Can you work these out from the model? Positions are in its coordinate system, mm. Give positions to 0.01 mm unless a question says otherwise; leave off trailing zeros. Write each loop counter-clockwise with the first axis right and the second up, starting at its lowest first coordinate (ties: lowest second). Pieces come first, ordered by that corner, then holes. Notation, with made-up numbers: (45.5, -4.75) -> (69.5, -4.75) arc R24 cw to (69.5, 31.25) -> close; hole circle Ø3 at (11.5, 38). An arc over 180 degrees is marked (long way). One line per item, written item: value.
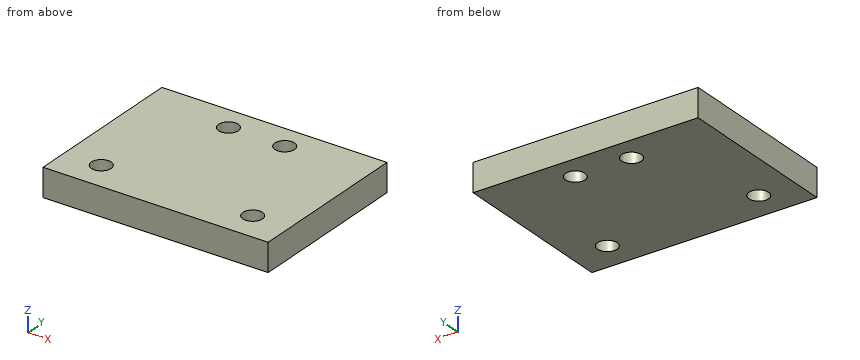
from build123d import *

# Parameters (mm, degrees)
SKETCH1_W           = 40
SKETCH1_H           = 30
SKETCH1_R           = 1.75
BOSS_EXTRUDE1_DEPTH = 5


with BuildPart() as part:
    # Sketch1 → Boss-Extrude1 (new body)
    with BuildSketch(Plane.XY):
        with Locations((20, 15)):
            Rectangle(SKETCH1_W, SKETCH1_H)
        with Locations((15, 25.5)):
            Circle(SKETCH1_R, mode=Mode.SUBTRACT)
        with Locations(Location((25, 25.5, 0), (0, 0, 180))):
            Circle(SKETCH1_R, mode=Mode.SUBTRACT)
        with Locations((6.55, 5.4)):
            Circle(SKETCH1_R, mode=Mode.SUBTRACT)
        with Locations(Location((33.45, 5.4, 0), (0, 0, 180))):
            Circle(SKETCH1_R, mode=Mode.SUBTRACT)
    extrude(amount=-BOSS_EXTRUDE1_DEPTH)


solid = part.part
1) If we section it at B-B (x = 33.45): Write out the boundary of the cut face in (y, z).
Answer list:
outline: (0, -5) -> (3.65, -5) -> (3.65, 0) -> (0, 0) -> close; (7.15, -5) -> (30, -5) -> (30, 0) -> (7.15, 0) -> close
2) If we section it at A-A (y = 5.4): Write out the boundary of the cut face in (x, z).
Answer list:
outline: (0, -5) -> (4.8, -5) -> (4.8, 0) -> (0, 0) -> close; (8.3, -5) -> (31.7, -5) -> (31.7, 0) -> (8.3, 0) -> close; (35.2, -5) -> (40, -5) -> (40, 0) -> (35.2, 0) -> close
3) If we section it at C-C (z = -3.3): Write out the boundary of the cut face in (x, y).
Answer list:
outline: (0, 0) -> (40, 0) -> (40, 30) -> (0, 30) -> close; hole circle Ø3.5 at (6.55, 5.4); hole circle Ø3.5 at (15, 25.5); hole circle Ø3.5 at (25, 25.5); hole circle Ø3.5 at (33.45, 5.4)
4) I need wall thicknesses on L1, parallel to X at y = 5.5, z = -1.5; L2, parallel to Y at x = 15, z = -1.2; L3, parallel to X at y = 4.25, z = -2.05. Which ranges of each line are inside material? Lowest first, please.
Answer list:
L1: x = 0 to 4.8, 8.3 to 31.7, 35.2 to 40
L2: y = 0 to 23.75, 27.25 to 30
L3: x = 0 to 5.23, 7.87 to 32.13, 34.77 to 40
